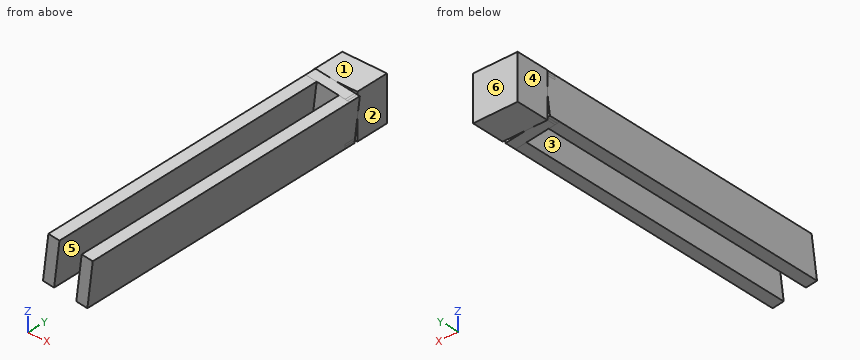
from build123d import *

# Parameters (mm, degrees)
F0_W     = 100
F0_H     = 100
F1_DEPTH = 75
F3_DEPTH = 25
F5_DEPTH = 650


# Not quite as in the source:
# - a feature names something its author has since deleted; it is built from what else it names


with BuildPart() as f1:
    # F0 (on Front) → F1 (new body)
    with BuildSketch(Plane.XZ):
        with Locations((50, 50)):
            Rectangle(F0_W, F0_H)
    extrude(amount=F1_DEPTH)

    # F2 (on face) → F3 (join)
    with BuildSketch(Plane.XZ.offset(75)):
        Polygon((100, 94.3057966884), (100, 46.974800806), (105.6538372319, 93.6205058254), align=None)
        Polygon((94.9213680166, 94.9213680166), (50, 50), (94.9217934551, 5.0782065449), (100, 46.974800806), (100, 94.3057966884), align=None)
        Polygon((0, 53.0131088143), (-5.6523319044, 6.3798231584), (0, 5.6947147534), align=None)
        Polygon((6.3804113302, 105.6532490601), (5.6951917585, 100), (53.0212637714, 100), align=None)
        Polygon((94.3062736934, 0), (46.9829557631, 0), (93.6210939972, -5.6529200762), align=None)
        Polygon((5.6951917585, 100), (5.0795135743, 94.9204864257), (50, 50), (94.9213680166, 94.9213680166), (53.0212637714, 100), align=None)
        Polygon((50, 50), (5.0790881358, 5.0790881358), (46.9829557631, 0), (94.3062736934, 0), (94.9217934551, 5.0782065449), align=None)
        Polygon((5.0795135743, 94.9204864257), (0, 53.0131088143), (0, 5.6947147534), (5.0790881358, 5.0790881358), (50, 50), align=None)
    extrude(amount=F3_DEPTH)

    # F4 (on face) → F5 (join)
    with BuildSketch(Plane.XZ.offset(100)):
        Polygon((31.1987678056, 102.6450632514), (6.3804113302, 105.6532490601), (-5.6523319044, 6.3798231584), (19.166024571, 3.3716373498), align=None)
        Polygon((93.6210939972, -5.6529200762), (105.6538372319, 93.6205058254), (80.8354807565, 96.6286916341), (68.8027375218, -2.6447342676), align=None)
    extrude(amount=F5_DEPTH)


solid = f1.part
Could you check a few things on this model? Use its own coordinates, in mm. Face numbers are marked on the shaded views. A direction names the side the tool comes from. Give positions to 0.01 mm unless a question says otherwise; leave off trailing zeros. Loops run counter-clockwise (first coordinate to the right, second up) from the corner with the lowest first, then second, coordinate; pieces in that order, holes last. Notation, with made-up numbers: (-34.75, -9.5) -> (10.25, -9.5) arc R22 cw to (10.25, 26.5) -> close; hole circle Ø11 at (47.5, 68). An arc over 180 degrees is marked (long way). Return JSON: item names as keys, results as strings.
Item 1: I'm going to push flat-ended pins straight in: pin 1 (10 mm diameter, centred on x = 9, y = -572.5, fed in from -Z); pin 2 (3 mm diameter, centred on x = 9.5, y = -260, fed in from +Z); pin 3 (4 mm diameter, centred on x = 60, y = -98.5, fed in from -Z); pin 4 (6 mm diameter, centred on x = 34.5, z = 102, fed in from +Y). Where does each tip first touch, or does it pass through?
Geometry results:
{"pin 1": "stops at z = 4", "pin 2": "stops at z = 105.46", "pin 3": "stops at z = -1.82", "pin 4": "stops at y = 0"}
Item 2: Which directions (+Z, -Z, +X, -X, +Y, -Y) give clear straight access to the entire face, cutting with the end or side of a thin tool? Please do the marked faces 1, 2 and 3.
Geometry results:
{"face 1": "+Z, +X, -X, +Y", "face 2": "+Z, -Z, +X, +Y", "face 3": "+Z, -Y"}
Item 3: If we section it at B-B on z = 85: List the corners of the cut face in (x, y) for me.
Geometry results:
{"outline": "(0, -75) -> (3.88, -75) -> (3.88, -750) -> (29.06, -750) -> (29.06, -100) -> (79.43, -100) -> (79.43, -750) -> (104.61, -750) -> (104.61, -75) -> (100, -75) -> (100, 0) -> (0, 0) -> close"}
Item 4: If we section it at A-A on y = -127: List the corners of the cut face in (x, z) for me, plus the area to 3 significant figures.
Geometry results:
{"outline": "(-5.65, 6.38) -> (19.17, 3.37) -> (31.2, 102.65) -> (6.38, 105.65) -> close; (68.8, -2.64) -> (93.62, -5.65) -> (105.65, 93.62) -> (80.84, 96.63) -> close", "area": "5,000 mm²"}
Item 5: We'd pull the mould along X, two halves only. Please class the marked faces 4, 5 and 6: +X half, -X half, draft (parallel to the pull), parting line (faces both ways), or undercut.
Geometry results:
{"face 4": "-X half", "face 5": "undercut", "face 6": "draft"}
Item 6: I need wall thicknesses on L1, parallel to Y at x = 46.5, z = 16; L2, parallel to X at y = -392, z = 9; L3, parallel to X at y = -565.5, z = 43. Which ranges of each line are inside material? Lowest first, please. Write a range as from..to.
Geometry results:
{"L1": "y = -100..0", "L2": "x = -5.33..19.85, 70.21..95.4", "L3": "x = -1.21..23.97, 74.34..99.52"}
